Work out the finished part from the listing and answer in its coordinate system (mm). Give positions to 0.01 mm unless a question says otherwise; leave off trailing zeros. Order: outer loops, then holes, each group sorted by start corner. A loop starts at its lowest first (then second) coordinate and runs counter-clockwise, first axis right, second up.
```python
from build123d import *

# Parameters (mm, degrees)
SKETCH1_R           = 3.175
SKETCH1_R_2         = 1.63195
BOSS_EXTRUDE1_DEPTH = 3.175
CUT_EXTRUDE1_DEPTH  = 6.499261314
CIRPATTERN1_COUNT   = 16


with BuildPart() as part:
    # Sketch1 → Boss-Extrude1 (new body)
    with BuildSketch(Plane(origin=(0, 0, 0), x_dir=(1, 0, 0), z_dir=(0, 1, 0))):
        with Locations(Location((0, 0, 0), (0, 0, 270))):
            Circle(SKETCH1_R)
        with Locations(Location((0, 0, 0), (0, 0, 270))):
            Circle(SKETCH1_R_2, mode=Mode.SUBTRACT)
    extrude(amount=BOSS_EXTRUDE1_DEPTH)

    # Sketch2 → Cut-Extrude1 (cut, through all)
    with BuildSketch(Plane(origin=(0, 3.175, 0), x_dir=(1, 0, 0), z_dir=(0, 1, 0))):
        with BuildLine():
            ThreePointArc((-0.1524, 3.171340291), (-0.226750807, 2.98179915), (-0.241694661, 2.778746034))
            ThreePointArc((-0.241694661, 2.778746034), (-0.25338078, 2.575323775), (-0.318555556, 2.382270856))
            ThreePointArc((-0.318555556, 2.382270856), (-0.468894712, 2.357292902), (-0.61734863, 2.322837219))
            ThreePointArc((-0.61734863, 2.322837219), (-0.751440425, 2.476253552), (-0.84008332, 2.659719129))
            ThreePointArc((-0.84008332, 2.659719129), (-0.931594704, 2.841596982), (-1.072820147, 2.98825734))
            ThreePointArc((-1.072820147, 2.98825734), (-0.619411772, 3.113993265), (-0.1524, 3.171340291))
        make_face()
    cut_extrude1 = extrude(amount=-CUT_EXTRUDE1_DEPTH, mode=Mode.SUBTRACT)

    # CirPattern1: Cut-Extrude1 ×16 about axis
    cirpattern1_axis = Axis((0, 0, 0), (0, 1, 0))
    for i in range(1, CIRPATTERN1_COUNT):
        add(cut_extrude1.rotate(cirpattern1_axis, i * 360 / CIRPATTERN1_COUNT), mode=Mode.SUBTRACT)


solid = part.part
```
1. The mould has two halves that part along X. Classify faces 1 (the face through (0, 0, 2)), 2 (the face through (-1.593, 1.565, -0.354)): pulls with the +X half, pulls with the -X half, needs draft (parallel to the pull), parting line crosses it, or undercut.
Findings below:
face 1: needs draft
face 2: undercut
2. The part is cut by section A-A (z = 0). Write down the section's boundary in (x, y) (3 decimals).
Findings below:
outline: (-3.175, 0) - (-1.632, 0) - (-1.632, 3.175) - (-3.175, 3.175) - close; (1.632, 0) - (3.175, 0) - (3.175, 3.175) - (1.632, 3.175) - close
3. The part is cut by section B-B (x = 0). Write down the section's boundary in (y, z) (3 decimals).
Findings below:
outline: (0, -3.175) - (3.175, -3.175) - (3.175, -1.632) - (0, -1.632) - close; (0, 1.632) - (3.175, 1.632) - (3.175, 3.175) - (0, 3.175) - close
4. Straight lines are drawn through the part: probe 1 along X at (y, z) = (2.2, 2); probe 2 along Z at (x, y) = (2.5, 0.95). For each, find the intervals that lie inside material, in ascending order.
Findings below:
probe 1: x = -2.3 to -1.64, -1.33 to 1.33, 1.64 to 2.3
probe 2: z = -1.3 to -0.77, -0.27 to 0.27, 0.77 to 1.3
